Work out the finished part from the listing and answer in its coordinate system (mm). A direction names the side the tool comes from. Round coordinates to 2 decimals unless told otherwise and drop trailing zeros. Write each loop counter-clockwise with the first axis right and the second up, starting at its lowest first coordinate (ties: lowest second). Pieces come first, ordered by that corner, then holes.
1. Find section A-A (y = 10.7). Count the separate pieces of the cut face and the enclosed holes in it, and give its area (3 significant figures).
2. Determine the mould class of faces 5 (the face through (-10.29, 7.47, 36.52)), 6 (the face through (-1, 22, 38)) for opening direction X: pulls with the +X half, pulls with the -X half, needs draft (parallel to the pull), parting line crosses it, or undercut.
3. Find section D-D (x = 3.5). Write down the section's boundary in (y, z), and give its area (3 significant figures).
4. Find section C-C (y = 23.75). Write down the section's boundary in (x, z) (3 decimals).
5. A tool of negligible diameter and unlimited length cuts with its end or side. For faces 1 (the face through (-14, 11, 30.2)), 2 (the face through (-40.043, 1.331, 35.812)), 3 (the face through (-39.17, 14.38, -34.92)), 4 (the face through (5.575, 18, -37)), from which of +Z, -Z, +X, -X, +Y, -Y can it reach the whole face along a straight path? Write none if from no direction.
6. Straight lines are drawn through the part: probe 1 along X at (y, z) = (8.75, 7.5); probe 2 along Z at (x, y) = (38.5, 4); probe 3 along Z at (x, y) = (-28.5, 23.75). For each, find the intervals that lie inside material, in ascending order.
7. Find section B-B (z = 27.5). Write down the section's boundary in (x, y).
8. Flat-ended cylindrical pins translate along their axes: pin 1 Ø2.5 at (x, z) = (14, 32) entering from +Y; pin 2 Ø4 at (x, z) = (13.5, 4.5) entering from +Y; pin 3 Ø3 at (x, z) = (-38.7, 33.44) entering from -Y; pin 4 Ø0.5 at (x, z) = (8.5, 25.5) entering from +Y. Find the tip coordinate at first contact, or state that the pin passes through.
```python
from build123d import *

# Parameters (mm, degrees)
SKETCH2_W            = 70
SKETCH2_H            = 70
BOSS_EXTRUDE1_DEPTH  = 2
BOSS_EXTRUDE2_DEPTH  = 18
SKETCH3_3_W          = 1
SKETCH3_3_H          = 15
BOSS_EXTRUDE3_DEPTH  = 2.5
SKETCH4_W            = 72
SKETCH4_H            = 76
SKETCH4_W_2          = 70
SKETCH4_H_2          = 70
BOSS_EXTRUDE4_DEPTH  = 26.4
SKETCH12_R           = 1.55
BOSS_EXTRUDE10_DEPTH = 26.4
BOSS_EXTRUDE11_DEPTH = 5
SKETCH1_R            = 1.18
SKETCH1_R_2          = 1.6
CUT_EXTRUDE1_DEPTH   = 25
FILLET1_R            = 3
CUT_EXTRUDE4_DEPTH   = 2.7
CUT_EXTRUDE5_DEPTH   = 10


with BuildPart() as part:
    # Sketch2 → Boss-Extrude1 (new body)
    with BuildSketch(Plane(origin=(0, 0, 0), x_dir=(1, 0, 0), z_dir=(0, 1, 0))):
        Rectangle(SKETCH2_W, SKETCH2_H)
    extrude(amount=BOSS_EXTRUDE1_DEPTH)

    # Sketch3 → Boss-Extrude2 (add)
    with BuildSketch(Plane(origin=(0, 2, 0), x_dir=(1, 0, 0), z_dir=(0, 1, 0))):
        Polygon((13.05, -31.2), (14.15, -31.2), (14.15, -35), (15.15, -35), (15.15, -30.2), (13.05, -30.2), align=None)
        Polygon((-15.15, -35), (-14.15, -35), (-14.15, -31.2), (-13.05, -31.2), (-13.05, -30.2), (-15.15, -30.2), align=None)
    extrude(amount=BOSS_EXTRUDE2_DEPTH)

    # Sketch3<3> → Boss-Extrude3 (add)
    with BuildSketch(Plane(origin=(0, 2, 0), x_dir=(1, 0, 0), z_dir=(0, 1, 0))):
        with Locations((-8.3, -27.5)):
            Rectangle(SKETCH3_3_W, SKETCH3_3_H)
        with Locations((8.3, -27.5)):
            Rectangle(SKETCH3_3_W, SKETCH3_3_H)
    extrude(amount=BOSS_EXTRUDE3_DEPTH)

    # Sketch4 → Boss-Extrude4 (add)
    with BuildSketch(Plane(origin=(0, 0, 0), x_dir=(1, 0, 0), z_dir=(0, 1, 0))):
        Rectangle(SKETCH4_W, SKETCH4_H)
        Rectangle(SKETCH4_W_2, SKETCH4_H_2, mode=Mode.SUBTRACT)
    extrude(amount=BOSS_EXTRUDE4_DEPTH)

    # Sketch12 → Boss-Extrude10 (add)
    # profile 1 of 2: a face of its own
    with BuildSketch(Plane(origin=(0, 0, 0), x_dir=(1, 0, 0), z_dir=(0, 1, 0))):
        with BuildLine():
            Line((36, -38), (42.4, -38))
            Line((42.4, -38), (42.4, 38))
            Line((42.4, 38), (36, 38))
            Line((36, 38), (36, 35.746040388))
            ThreePointArc((36, 35.746040388), (35.639428233, 31.642432378), (39.4, 29.960852562))
            Line((39.4, 29.960852562), (39.4, -29.960852562))
            ThreePointArc((39.4, -29.960852562), (35.639428233, -31.642432378), (36, -35.746040388))
            Line((36, -35.746040388), (36, -38))
        make_face()
        with Locations(Location((38.7, -33.441154273, 0), (0, 0, 270))):
            Circle(SKETCH12_R, mode=Mode.SUBTRACT)
        with Locations(Location((38.7, 33.441154273, 0), (0, 0, 270))):
            Circle(SKETCH12_R, mode=Mode.SUBTRACT)
    # profile 2 of 2: a face of its own
    with BuildSketch(Plane(origin=(0, 0, 0), x_dir=(1, 0, 0), z_dir=(0, 1, 0))):
        with BuildLine():
            Line((-36, 38), (-36, 35.746040388))
            ThreePointArc((-36, 35.746040388), (-35.639428233, 31.642432378), (-39.4, 29.960852562))
            Line((-39.4, 29.960852562), (-39.4, -29.960852562))
            ThreePointArc((-39.4, -29.960852562), (-35.639428233, -31.642432378), (-36, -35.746040388))
            Line((-36, -35.746040388), (-36, -38))
            Line((-36, -38), (-42.4, -38))
            Line((-42.4, -38), (-42.4, 38))
            Line((-42.4, 38), (-36, 38))
        make_face()
        with Locations(Location((-38.7, 33.441154273, 0), (0, 0, 90))):
            Circle(SKETCH12_R, mode=Mode.SUBTRACT)
        with Locations(Location((-38.7, -33.441154273, 0), (0, 0, 90))):
            Circle(SKETCH12_R, mode=Mode.SUBTRACT)
    extrude(amount=BOSS_EXTRUDE10_DEPTH)

    # Sketch13 → Boss-Extrude11 (add)
    with BuildSketch(Plane(origin=(0, 0, 0), x_dir=(1, 0, 0), z_dir=(0, 1, 0))):
        with BuildLine():
            Line((39.4, 29.960852562), (39.4, -29.960852562))
            ThreePointArc((39.4, -29.960852562), (37.540086013, -30.085994136), (36, -31.136268159))
            Line((36, -31.136268159), (36, 31.136268159))
            ThreePointArc((36, 31.136268159), (37.540086013, 30.085994136), (39.4, 29.960852562))
        make_face()
        with BuildLine():
            Line((-39.4, -29.960852562), (-39.4, 29.960852562))
            ThreePointArc((-39.4, 29.960852562), (-37.540086013, 30.085994136), (-36, 31.136268159))
            Line((-36, 31.136268159), (-36, -31.136268159))
            ThreePointArc((-36, -31.136268159), (-37.540086013, -30.085994136), (-39.4, -29.960852562))
        make_face()
    extrude(amount=BOSS_EXTRUDE11_DEPTH)

    # Sketch1 → Cut-Extrude1 (cut)
    # profile 1 of 5: a face of its own
    with BuildSketch(Plane.XY.offset(38)):
        with BuildLine():
            ThreePointArc((6.310018649, 16.760020721), (0, 21.7), (-6.310018649, 16.760020721))
            ThreePointArc((-6.310018649, 16.760020721), (-10.201264735, 7.325560023), (0, 7.033939444))
            ThreePointArc((0, 7.033939444), (10.201264735, 7.325560023), (6.310018649, 16.760020721))
        make_face()
        with BuildLine():
            ThreePointArc((4.487784147, 14.868649052), (0, 19.7), (-4.487784147, 14.868649052))
            ThreePointArc((-4.487784147, 14.868649052), (-8.121835414, 7.890348127), (-0.800613643, 10.771792937))
            ThreePointArc((-0.800613643, 10.771792937), (0, 10.7), (0.800613643, 10.771792937))
            ThreePointArc((0.800613643, 10.771792937), (8.121835414, 7.890348127), (4.487784147, 14.868649052))
        make_face(mode=Mode.SUBTRACT)
    # profile 2 of 5: a face of its own
    with BuildSketch(Plane.XY.offset(38)):
        with BuildLine():
            ThreePointArc((0.800613643, 10.771792937), (8.121835414, 7.890348127), (4.487784147, 14.868649052))
            ThreePointArc((4.487784147, 14.868649052), (0, 19.7), (-4.487784147, 14.868649052))
            ThreePointArc((-4.487784147, 14.868649052), (-8.121835414, 7.890348127), (-0.800613643, 10.771792937))
            ThreePointArc((-0.800613643, 10.771792937), (0, 10.7), (0.800613643, 10.771792937))
        make_face()
        with Locations((-5, 10.7)):
            Circle(SKETCH1_R, mode=Mode.SUBTRACT)
        with Locations((5, 10.7)):
            Circle(SKETCH1_R, mode=Mode.SUBTRACT)
        with Locations((0, 15.2)):
            Circle(SKETCH1_R_2, mode=Mode.SUBTRACT)
    # profile 3 of 5: a face of its own
    with BuildSketch(Plane.XY.offset(38)):
        with Locations((0, 15.2)):
            Circle(SKETCH1_R_2)
    # profile 4 of 5: a face of its own
    with BuildSketch(Plane.XY.offset(38)):
        with Locations((5, 10.7)):
            Circle(SKETCH1_R)
    # profile 5 of 5: a face of its own
    with BuildSketch(Plane.XY.offset(38)):
        with Locations((-5, 10.7)):
            Circle(SKETCH1_R)
    extrude(amount=-CUT_EXTRUDE1_DEPTH, mode=Mode.SUBTRACT)

    # Fillet1
    fillet1_edges = [part.edges().sort_by_distance(p)[0] for p in [
        (42.4, 13.2, -38),
        (42.4, 13.2, 38),
        (-42.4, 13.2, 38),
        (-42.4, 13.2, -38),
    ]]
    fillet(fillet1_edges, radius=FILLET1_R)

    # Sketch14 → Cut-Extrude4 (cut)
    with BuildSketch(Plane.XZ):
        Polygon((-41.425, 31.86787479), (-38.7, 30.294595306), (-35.975, 31.86787479), (-35.975, 35.014433757), (-38.7, 36.58771324), (-41.425, 35.014433757), align=None)
        Polygon((41.425, 31.86787479), (41.425, 35.014433757), (38.7, 36.58771324), (35.975, 35.014433757), (35.975, 31.86787479), (38.7, 30.294595306), align=None)
        Polygon((41.425, -35.014433757), (41.425, -31.86787479), (38.7, -30.294595306), (35.975, -31.86787479), (35.975, -35.014433757), (38.7, -36.58771324), align=None)
        Polygon((-35.975, -35.014433757), (-35.975, -31.86787479), (-38.7, -30.294595306), (-41.425, -31.86787479), (-41.425, -35.014433757), (-38.7, -36.58771324), align=None)
    extrude(amount=-CUT_EXTRUDE4_DEPTH, mode=Mode.SUBTRACT)

    # Sketch15 → Cut-Extrude5 (cut)
    with BuildSketch(Plane(origin=(0, 0, -38), x_dir=(-1, 0, 0), z_dir=(0, 0, -1))):
        Polygon((-5.575, 14), (-5.575, 26.4), (5.575, 26.4), (5.575, 14), (5.575, 8.5), (-5.575, 8.5), align=None)
    extrude(amount=-CUT_EXTRUDE5_DEPTH, mode=Mode.SUBTRACT)


solid = part.part
```
Worked answers:
1. separate pieces: 2
1. enclosed holes: 6
1. area: 1,010 mm2
2. face 5: undercut
2. face 6: needs draft
3. outline: (0, -38) - (8.5, -38) - (8.5, -35) - (2, -35) - (2, 35) - (4.68, 35) - (4.68, 38) - (0, 38) - close; (20.68, 35) - (26.4, 35) - (26.4, 38) - (20.68, 38) - close
3. area: 197 mm2
4. outline: (-42.4, -35) arc R3 ccw to (-39.4, -38) - (-5.575, -38) - (-5.575, -35) - (-35, -35) - (-35, 35) - (35, 35) - (35, -35) - (5.575, -35) - (5.575, -38) - (39.4, -38) arc R3 ccw to (42.4, -35) - (42.4, 35) arc R3 ccw to (39.4, 38) - (-39.4, 38) arc R3 ccw to (-42.4, 35) - close; hole circle Ø3.1 at (-38.7, -33.441); hole circle Ø3.1 at (-38.7, 33.441); hole (-39.4, -29.961) arc R3.55 cw to (-36, -31.136) - (-36, 31.136) arc R3.55 cw to (-39.4, 29.961) - close; hole (36, -31.136) arc R3.55 cw to (39.4, -29.961) - (39.4, 29.961) arc R3.55 cw to (36, 31.136) - close; hole circle Ø3.1 at (38.7, -33.441); hole circle Ø3.1 at (38.7, 33.441)
5. face 1: +Y
5. face 2: -Y
5. face 3: +Y, -Y
5. face 4: -Z, +Y
6. probe 1: x = -42.4 to -39.4, -36 to -35, 35 to 36, 39.4 to 42.4
6. probe 2: z = -38 to -34.98, -31.9 to 31.9, 34.98 to 38
6. probe 3: z = -38 to -35, 35 to 38
7. outline: (-42.4, 0) - (42.4, 0) - (42.4, 26.4) - (39.4, 26.4) - (39.4, 5) - (36, 5) - (36, 26.4) - (35, 26.4) - (35, 2) - (8.8, 2) - (8.8, 4.5) - (7.8, 4.5) - (7.8, 2) - (-7.8, 2) - (-7.8, 4.5) - (-8.8, 4.5) - (-8.8, 2) - (-35, 2) - (-35, 26.4) - (-36, 26.4) - (-36, 5) - (-39.4, 5) - (-39.4, 26.4) - (-42.4, 26.4) - close
8. pin 1: stops at y = 20
8. pin 2: stops at y = 2
8. pin 3: passes through
8. pin 4: stops at y = 4.5
